The model under review builds one solid part; all positions refer to its coordinate system, in mm. A direction names the side the tool comes from. Round coordinates to 2 decimals unless told otherwise and drop trailing zeros. Write each loop counter-clockwise with the first axis right and the second up, starting at its lowest first coordinate (ties: lowest second). Pieces come first, ordered by that corner, then holes. Notation, with made-up numbers: (5, 48.25) - (21, 48.25) arc R24 ccw to (21, 84.25) - close; hole circle Ø1 at (37.5, -29). An arc over 180 degrees is marked (long way). Use one line per item in the form item = value.
from build123d import *

# Parameters (mm, degrees)
SKETCH1_W           = 26
SKETCH1_H           = 19
BOSS_EXTRUDE1_DEPTH = 1.6
SKETCH2_W           = 8.95
SKETCH2_H           = 6.85
BOSS_EXTRUDE2_DEPTH = 3.2
SKETCH3_R           = 0.45
CUT_EXTRUDE1_DEPTH  = 2.6
SKETCH4_R           = 1.2
CUT_EXTRUDE2_DEPTH  = 2.6
SKETCH5_R           = 0.45
CUT_EXTRUDE3_DEPTH  = 2.6
SKETCH6_W           = 2
SKETCH6_H           = 2
SKETCH6_W_2         = 3
SKETCH6_H_2         = 2.3
CUT_EXTRUDE4_DEPTH  = 0.1
FILLET1_R           = 0.9
SKETCH8_W           = 2.5
SKETCH8_H           = 4.25
BOSS_EXTRUDE3_DEPTH = 1.95
SKETCH9_W           = 1.95
SKETCH9_H           = 0.95
BOSS_EXTRUDE4_DEPTH = 1
SKETCH10_W          = 0.85
SKETCH10_H          = 1.4
BOSS_EXTRUDE5_DEPTH = 0.55
LPATTERN1_COUNT     = 4
LPATTERN1_PITCH     = 1.85
SKETCH11_W          = 0.2
SKETCH11_H          = 1.95
CUT_EXTRUDE5_DEPTH  = 0.01


with BuildPart() as part:
    # Sketch1 → Boss-Extrude1 (new body)
    with BuildSketch(Plane(origin=(0, 0, 0), x_dir=(1, 0, 0), z_dir=(0, 1, 0))):
        Rectangle(SKETCH1_W, SKETCH1_H)
    extrude(amount=BOSS_EXTRUDE1_DEPTH)

    # Sketch2 → Boss-Extrude2 (add)
    with BuildSketch(Plane(origin=(0, 1.6, 0), x_dir=(1, 0, 0), z_dir=(0, 1, 0))):
        with Locations((5.025, 6.945)):
            Rectangle(SKETCH2_W, SKETCH2_H)
    extrude(amount=BOSS_EXTRUDE2_DEPTH)

    # Sketch3 → Cut-Extrude1 (cut, through all)
    with BuildSketch(Plane(origin=(0, 1.6, 0), x_dir=(1, 0, 0), z_dir=(0, 1, 0))):
        with Locations((-10, -8.25)):
            Circle(SKETCH3_R)
        with Locations((7, -8.25)):
            Circle(SKETCH3_R)
    extrude(amount=-CUT_EXTRUDE1_DEPTH, mode=Mode.SUBTRACT)

    # Sketch4 → Cut-Extrude2 (cut, through all)
    with BuildSketch(Plane(origin=(0, 1.6, 0), x_dir=(1, 0, 0), z_dir=(0, 1, 0))):
        with Locations((-13.2, 3.9)):
            Circle(SKETCH4_R)
        with Locations((13.2, 3.9)):
            Circle(SKETCH4_R)
    extrude(amount=-CUT_EXTRUDE2_DEPTH, mode=Mode.SUBTRACT)

    # Sketch5 → Cut-Extrude3 (cut, through all)
    with BuildSketch(Plane(origin=(0, 1.6, 0), x_dir=(1, 0, 0), z_dir=(0, 1, 0))):
        with Locations((-11.95, 8.35)):
            Circle(SKETCH5_R)
        with Locations((11.95, 8.35)):
            Circle(SKETCH5_R)
    extrude(amount=-CUT_EXTRUDE3_DEPTH, mode=Mode.SUBTRACT)

    # Sketch6 → Cut-Extrude4 (cut)
    with BuildSketch(Plane(origin=(0, 1.6, 0), x_dir=(1, 0, 0), z_dir=(0, 1, 0))):
        with Locations((-12, 8.5)):
            Rectangle(SKETCH6_W, SKETCH6_H)
        with Locations((12, 8.5)):
            Rectangle(SKETCH6_W, SKETCH6_H)
        with Locations((-10, -8.25)):
            Rectangle(SKETCH6_W_2, SKETCH6_H_2)
        with Locations((7, -8.25)):
            Rectangle(SKETCH6_W_2, SKETCH6_H_2)
    extrude(amount=-CUT_EXTRUDE4_DEPTH, mode=Mode.SUBTRACT)

    # Fillet1
    fillet1_edges = [part.edges().sort_by_distance(p)[0] for p in [
        (0.55, 1.6, -9.935),
        (9.5, 1.6, -9.935),
        (0.55, 4.8, -6.945),
        (9.5, 4.8, -6.945),
    ]]
    fillet(fillet1_edges, radius=FILLET1_R)

    # Sketch8 → Boss-Extrude3 (add)
    with BuildSketch(Plane(origin=(0, 1.6, 0), x_dir=(1, 0, 0), z_dir=(0, 1, 0))):
        with Locations((-11.75, -1.425)):
            Rectangle(SKETCH8_W, SKETCH8_H)
    extrude(amount=BOSS_EXTRUDE3_DEPTH)

    # Sketch9 → Boss-Extrude4 (add)
    with BuildSketch(Plane.ZY.offset(13)):
        with Locations((1.425, 2.575)):
            Rectangle(SKETCH9_W, SKETCH9_H)
    extrude(amount=BOSS_EXTRUDE4_DEPTH)

    # Sketch10 → Boss-Extrude5 (add)
    with BuildSketch(Plane(origin=(0, 1.6, 0), x_dir=(1, 0, 0), z_dir=(0, 1, 0))):
        with Locations((-9.675, 8)):
            Rectangle(SKETCH10_W, SKETCH10_H)
    boss_extrude5 = extrude(amount=BOSS_EXTRUDE5_DEPTH)

    # LPattern1: Boss-Extrude5 ×4
    with Locations(*[(i * LPATTERN1_PITCH, 0, 0) for i in range(1, LPATTERN1_COUNT)]):
        add(boss_extrude5)

    # Sketch11 → Cut-Extrude5 (cut)
    with BuildSketch(Plane(origin=(0, 3.05, 0), x_dir=(1, 0, 0), z_dir=(0, 1, 0))):
        with Locations((-13.9, -1.425)):
            Rectangle(SKETCH11_W, SKETCH11_H)
    extrude(amount=-CUT_EXTRUDE5_DEPTH, mode=Mode.SUBTRACT)


solid = part.part
(1) Add section B-B on z = -6. Write out the cut boundary in (x, y), then the cut area to 3 significant figures.
Geometry results:
outline = (-13, 0) - (13, 0) - (13, 1.6) - (9.5, 1.6) - (9.5, 3.9) arc R0.9 ccw to (8.6, 4.8) - (1.45, 4.8) arc R0.9 ccw to (0.55, 3.9) - (0.55, 1.6) - (-13, 1.6) - close
area = 69.9 mm2
(2) Insertion check: P1, Ø1.5, axis at x = 4, y = 2.5, coming from the +Z side; P2, Ø1, axis at x = 9, z = -8, coming from the -Y side; P3, Ø1.2, axis at y = 3, z = -6.5, coming from the +X side; P4, Ø9.5, axis at x = -5.5, z = -4, coming from the +Y side. Each pin has a flat end and moves straight along its axis. Give the tip position at first contact, or say it passes through.
Geometry results:
P1 = -3.52
P2 = 0
P3 = 9.5
P4 = 2.15
(3) To check wall thickness, follow L1, parallel to X at y = 0.6, z = 8.25; L2, parallel to X at y = 0.85, z = -8.35; L3, parallel to Z at x = -11.95, y = 1.2. State the ranges of each line that lie inside material, in increasing order.
Geometry results:
L1 = -13 to -10.45, -9.55 to 6.55, 7.45 to 13
L2 = -13 to -12.4, -11.5 to 11.5, 12.4 to 13
L3 = -9.5 to -8.8, -7.9 to 9.5
(4) The part is to be moulded in two halves that separate along X. For faces 4 (the flat face through (-13.5, 2.1, 1.4)), 5 (the cylindrical face through (7.429, 0.76, 8.115)), 6 (the cylindrical face through (9.23, 4.54, -6.99)), say which applies: +X half, -X half, draft (parallel to the pull), parting line (faces both ways), or undercut.
Geometry results:
face_4 = draft
face_5 = undercut
face_6 = +X half
(5) Add section D-D on z = -8.35. Count the separate pieces of the cut face and the enclosed holes in it, then the cut area to 3 significant figures.
Geometry results:
separate_pieces = 3
enclosed_holes = 0
area = 68.7 mm2
(6) Add section C-C on x = -7. Write out the cut boundary in (y, z), then the cut area to 3 significant figures.
Geometry results:
outline = (0, -9.5) - (1.6, -9.5) - (1.6, 9.5) - (0, 9.5) - close
area = 30.4 mm2
(7) Machinability: for faces 1 (the flat face through (-10.5, 3, 1)), 2 (the flat face through (-13.5, 2.6, 2.4)), 3 (the flat face through (-13.4, 3.05, 1.4)), which of the approach directions +Z, -Z, +X, -X, +Y, -Y give a long, thin tool a straight path to every point of the face, cutting with its end or side? Answer none if there is none.
Geometry results:
face_1 = +Z, -Z, +X, +Y
face_2 = +Z, -X, +Y, -Y
face_3 = +Z, -Z, -X, +Y
(8) Add section A-A on z = 8.25. Write out the cut boundary in (x, y).
Geometry results:
outline = (-13, 0) - (-10.45, 0) - (-10.45, 1.5) - (-11.5, 1.5) - (-11.5, 1.6) - (-13, 1.6) - close; (-9.55, 0) - (6.55, 0) - (6.55, 1.5) - (5.5, 1.5) - (5.5, 1.6) - (-8.5, 1.6) - (-8.5, 1.5) - (-9.55, 1.5) - close; (7.45, 0) - (13, 0) - (13, 1.6) - (8.5, 1.6) - (8.5, 1.5) - (7.45, 1.5) - close
